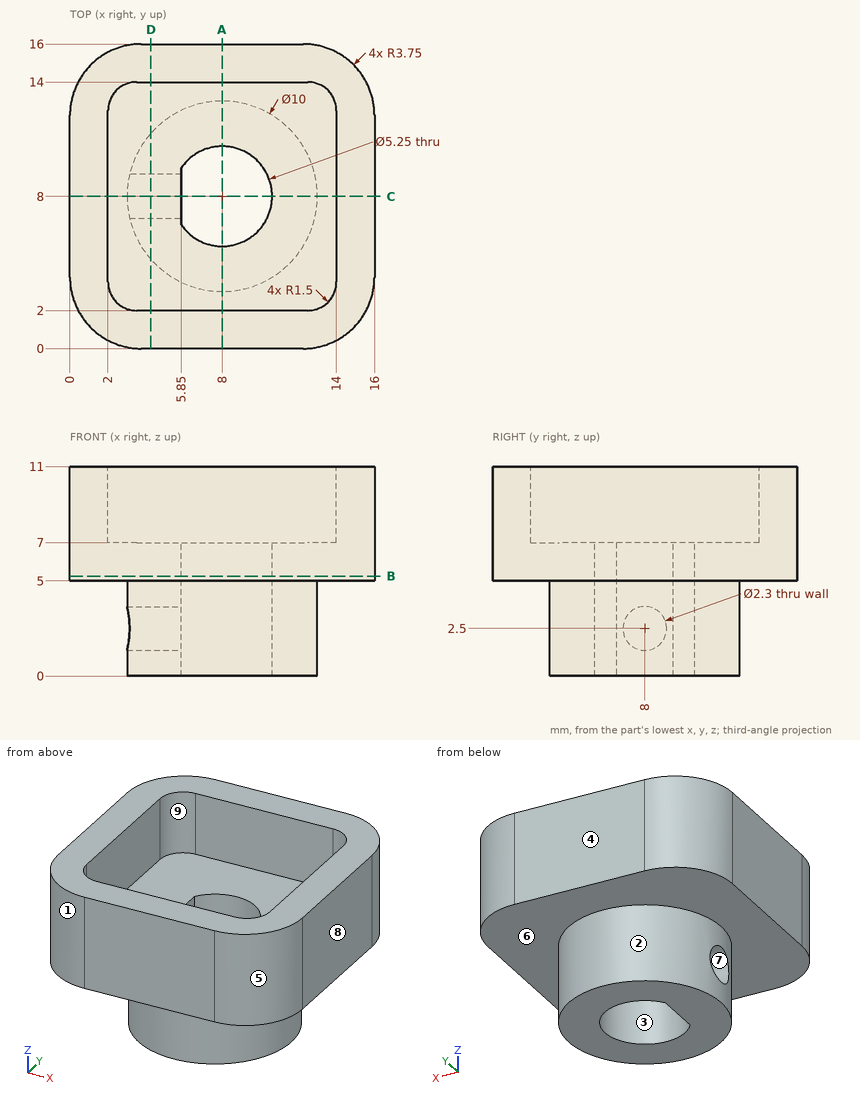
Could you check a few things on this drawing? It's one solid part, dimensions in mm from its lowest x, y, z. A direction names the side the tool comes from. Coordinates: 2 decimals unless noted, no trailing zeros. Order: outer loops, then holes, each group sorted by start corner. A loop starts at its lowest first (then second) coordinate and runs counter-clockwise, first axis right, second up.
1) Imagine slicing it at C-C on y = 8. List the corners of the cut face in (x, z) for me (3 decimals), and give its area (3 significant figures).
2) Imagine slicing it at B-B on z = 5.25. List the corners of the cut face in (x, y) for me (3 decimals).
3) Which directions (+Z, -Z, +X, -X, +Y, -Y) give clear straight access to the entire face, cutting with the end or side of a thin tool? Please do the marked faces 5, 6, 7, 8 and 9.
4) Will these pins go through, and if not, where does the flat tip stop? pin 1 (6 mm diameter, centred on x = 8, y = 8, fed in from +Z); pin 2 (2 mm diameter, centred on y = 8, z = 2.5, fed in from -X); pin 3 (3.5 mm diameter, centred on y = 8, z = 2.5, fed in from +X).
5) Imagine slicing it at A-A on x = 8. List the corners of the cut face in (y, z) for me (3 decimals), and give its area (4 significant figures).
6) We'd pull the mould along X, two halves only. Please class the marked faces 1, 2, 3 and 4: +X half, -X half, draft (parallel to the pull), parting line (faces both ways), or undercut.
7) I need wall thicknesses on line 1 (Y direction, x = 8, z = 3.75) (3 decimals); line 2 (Y direction, x = 12, z = 9.25); line 3 (Z direction, x = 5.25, y = 11.75). Which ranges of each line are inside material? Lowest first, please.
8) Imagine slicing it at D-D on x = 4.25. List the corners of the cut face in (y, z) for me.
Response values:
1. outline: (0, 5) - (3, 5) - (3, 3.65) - (5.85, 3.65) - (5.85, 7) - (2, 7) - (2, 11) - (0, 11) - close; (3, 0) - (5.85, 0) - (5.85, 1.35) - (3, 1.35) - close; (10.625, 0) - (13, 0) - (13, 5) - (16, 5) - (16, 11) - (14, 11) - (14, 7) - (10.625, 7) - close
1. area: 58.0 mm2
2. outline: (0, 3.75) arc R3.75 ccw to (3.75, 0) - (12.25, 0) arc R3.75 ccw to (16, 3.75) - (16, 12.25) arc R3.75 ccw to (12.25, 16) - (3.75, 16) arc R3.75 ccw to (0, 12.25) - close; hole (5.85, 6.494) arc R2.625 ccw (long way) to (5.85, 9.506) - close
3. face 5: +Z, -Z, +X, -Y
3. face 6: -Z
3. face 7: -X
3. face 8: +Z, -Z, +X, +Y, -Y
3. face 9: +Z
4. pin 1: stops at z = 7
4. pin 2: stops at x = 10.43
4. pin 3: stops at x = 13
5. outline: (0, 5) - (3, 5) - (3, 0) - (5.375, 0) - (5.375, 7) - (2, 7) - (2, 11) - (0, 11) - close; (10.625, 0) - (13, 0) - (13, 5) - (16, 5) - (16, 11) - (14, 11) - (14, 7) - (10.625, 7) - close
5. area: 61.25 mm2
6. face 1: -X half
6. face 2: parting line
6. face 3: undercut
6. face 4: draft
7. line 1: y = 3 to 5.375, 10.625 to 13
7. line 2: y = 0 to 2, 14 to 16
7. line 3: z = 0 to 7
8. outline: (0, 5) - (4.69, 5) - (4.69, 0) - (11.31, 0) - (11.31, 5) - (16, 5) - (16, 11) - (14, 11) - (14, 7) - (2, 7) - (2, 11) - (0, 11) - close; hole circle Ø2.3 at (8, 2.5)
